```python
from build123d import *

# Parameters (mm, degrees)
SKETCH_1_R          = 27.5
EXTRUDE_1_DEPTH     = 11
SKETCH_2_R          = 31
EXTRUDE_2_DEPTH     = 8
SKETCH_3_R          = 2.5
CUT_EXTRUDE_1_DEPTH = 15
SKETCH_4_R          = 15
CUT_EXTRUDE_2_DEPTH = 48.780749262
CHAMFER_1_SIZE      = 0.5
CHAMFER_2_SIZE      = 0.5


with BuildPart() as part:
    # 草图1 → 拉伸1 (new body)
    with BuildSketch(Plane.XY):
        Circle(SKETCH_1_R)
    extrude(amount=EXTRUDE_1_DEPTH)

    # 草图2 → 拉伸2 (add)
    with BuildSketch(Plane.XY.offset(11)):
        Circle(SKETCH_2_R)
    extrude(amount=EXTRUDE_2_DEPTH)

    # 草图3 → 切除-拉伸1 (cut)
    with BuildSketch(Plane.XY.offset(19)):
        with Locations((0, 22.5)):
            Circle(SKETCH_3_R)
        with Locations((15.909902577, 15.909902577)):
            Circle(SKETCH_3_R)
        with Locations((22.5, 0)):
            Circle(SKETCH_3_R)
        with Locations((15.909902577, -15.909902577)):
            Circle(SKETCH_3_R)
        with Locations((0, -22.5)):
            Circle(SKETCH_3_R)
        with Locations((-15.909902577, -15.909902577)):
            Circle(SKETCH_3_R)
        with Locations((-22.5, 0)):
            Circle(SKETCH_3_R)
        with Locations((-15.909902577, 15.909902577)):
            Circle(SKETCH_3_R)
    extrude(amount=-CUT_EXTRUDE_1_DEPTH, mode=Mode.SUBTRACT)

    # 草图4 → 切除-拉伸2 (cut, through all)
    with BuildSketch(Plane.XY.offset(19)):
        Circle(SKETCH_4_R)
    extrude(amount=-CUT_EXTRUDE_2_DEPTH, mode=Mode.SUBTRACT)

    # 倒角1
    chamfer_1_edges = [part.edges().sort_by_distance(p)[0] for p in [
        (-27.5, 0, 0),
        (-15, 0, 0),
        (-31, 0, 11),
        (-31, 0, 19),
    ]]
    chamfer(chamfer_1_edges, length=CHAMFER_1_SIZE)

    # 倒角2
    chamfer_2_edges = [part.edges().sort_by_distance(p)[0] for p in [
        (-15, 0, 19),
    ]]
    chamfer(chamfer_2_edges, length=CHAMFER_2_SIZE)


solid = part.part
```
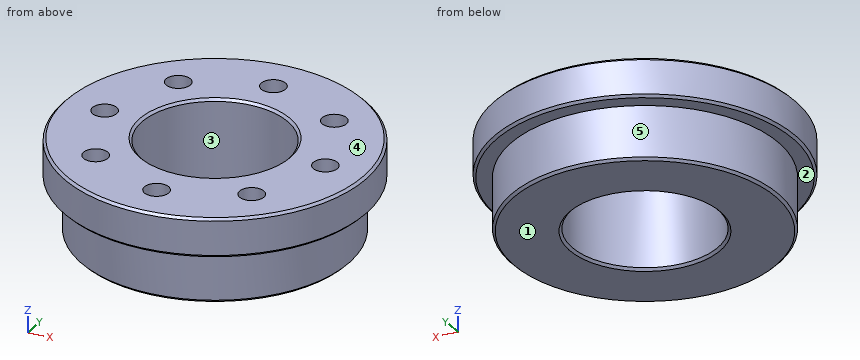
Geometry: final body of the model. Coordinates: model frame, mm. Face numbers are marked on the shaded views. A direction names the side the tool comes from. Coordinates: 2 decimals unless noted, no trailing zeros. Use CSV: the item, a comma, the result in double quotes.
1) Access query for the marked faces 1 and 2. Directions: +Z, -Z, +X, -X, +Y, -Y. A direction counts if a zero-diameter tool reaches every point of the face in a straight line with its end or side. Return the directions, or none.
Findings:
face 1,"-Z, +X, -X, +Y, -Y"
face 2,"-Z"
2) Mould query, pull axis Y, two halves, no side actions, for the marked faces 3, 4 and 5. Classes: +Y half, -Y half, draft (parallel to the pull), parting line (faces both ways), or undercut.
Findings:
face 3,"undercut"
face 4,"draft"
face 5,"parting line"
3) Pin query (flat end, axial travel): pin 1 Ø8 at (y, z) = (-7, 14) entering from -X; pin 2 Ø1.5 at (x, y) = (-23.5, -1) entering from +Z; pin 3 Ø2 at (y, z) = (21.5, 16.5) entering from -X; pin 4 Ø18 at (x, y) = (0, 0) entering from +Z. Return the tip coordinate at first contact, or that it passes through.
Findings:
pin 1,"stops at x = -30.85"
pin 2,"stops at z = 4"
pin 3,"stops at x = -23.25"
pin 4,"passes through"
4) Section C-C on z = 15.5. State how many separate pieces and enclosed holes the cut face has, then the cut area to 3 significant figures.
Findings:
separate pieces,"1"
enclosed holes,"9"
area,"2,160 mm^2"
5) Line query: line 1 (Y direction, x = 0, z = 8.25); line 2 (Y direction, x = -18, z = 14.25); line 3 (Y direction, x = -16.5, z = 7.25). Output: solid intervals per line, ascending.
Findings:
line 1,"y = -27.5 to -25, -20 to -15, 15 to 20, 25 to 27.5"
line 2,"y = -25.24 to -17.28, -14.54 to 14.54, 17.28 to 25.24"
line 3,"y = -22 to -18.34, -13.48 to 13.48, 18.34 to 22"
